Verification items for the finished model (mm, model axes). Face numbers are marked on the shaded views. A direction names the side the tool comes from. Round coordinates to 2 decimals unless told otherwise and drop trailing zeros. Order: outer loops, then holes, each group sorted by start corner. A loop starts at its lowest first (then second) coordinate and runs counter-clockwise, first axis right, second up. Notation, with made-up numbers: (51, 24.25) -> (85, 24.25) arc R38 cw to (85, 62.25) -> close; hole circle Ø3 at (81.5, 86.25). An arc over 180 degrees is marked (long way). Put each result on its own line as item: value.
```python
from build123d import *

# Parameters (mm, degrees)
SKETCH2_W          = 3.119119432
SKETCH2_H          = 0.920816202
CUT_EXTRUDE1_DEPTH = 7.874


with BuildPart() as part:
    # Sketch1 → Revolve1 (revolve)
    with BuildSketch(Plane.XY, mode=Mode.PRIVATE) as revolve1_sk:
        Polygon((0, 0), (12.7, 0), (12.7, 3.175), (1.905, 3.175), (0, 5.08), align=None)
    revolve(revolve1_sk.sketch.rotate(Axis((0, 0, 0), (1, 0, 0)), 90), axis=Axis((0, 0, 0), (1, 0, 0)))

    # Sketch2 → Cut-Extrude1 (cut, symmetric)
    with BuildSketch(Plane(origin=(0, 0, 0), x_dir=(1, 0, 0), z_dir=(0, 1, 0))):
        Rectangle(SKETCH2_W, SKETCH2_H)
    extrude(amount=CUT_EXTRUDE1_DEPTH, both=True, mode=Mode.SUBTRACT)


solid = part.part
```
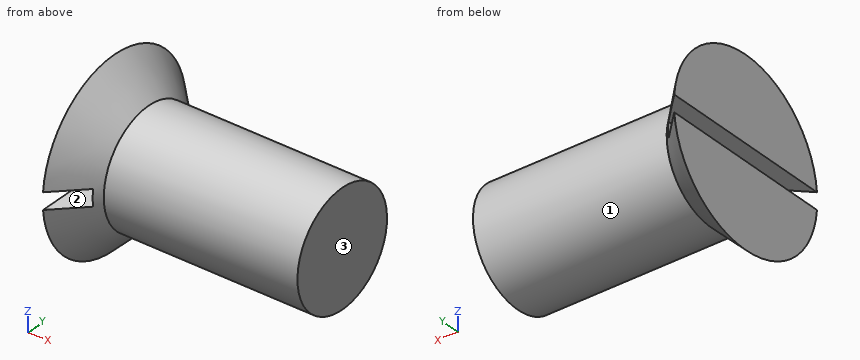
Item 1: Sectioned sample at C-C, the plane x = 1.75. Record the boundary of the cut face in (y, z), then the cut area to 3 significant figures.
Geometry check:
outline: circle Ø6.66 at (0, 0)
area: 34.8 mm2
Item 2: Tool access check on the marked faces 1, 2 and 3. Record the directions out of +Z, -Z, +X, -X, +Y, -Y that give a thin tool (end or side, any length) a straight path to the whole face; none if there is none.
Geometry check:
face 1: +X
face 2: -X, +Y, -Y
face 3: +Z, -Z, +X, +Y, -Y
Item 3: Sectioned sample at B-B, the plane z = 0. Record the boundary of the cut face in (x, y) (3 decimals), then the cut area to 3 significant figures.
Geometry check:
outline: (1.56, -3.52) -> (1.905, -3.175) -> (12.7, -3.175) -> (12.7, 3.175) -> (1.905, 3.175) -> (1.56, 3.52) -> close
area: 70.9 mm2
Item 4: Sectioned sample at A-A, the plane y = 0. Record the boundary of the cut face in (x, z) (3 decimals), then the cut area to 3 significant figures.
Geometry check:
outline: (0, -5.08) -> (1.905, -3.175) -> (12.7, -3.175) -> (12.7, 3.175) -> (1.905, 3.175) -> (0, 5.08) -> (0, 0.46) -> (1.56, 0.46) -> (1.56, -0.46) -> (0, -0.46) -> close
area: 82.8 mm2
Item 5: Depth check by flat-ended pin: pin 1 Ø0.7 at (y, z) = (-1, 0) entering from -X; pin 2 Ø1 at (x, y) = (4.5, 2.5) entering from +Z; pin 3 Ø4 at (y, z) = (1.5, -3.5) entering from -X; pin 4 Ø4 at (x, y) = (2, 1.5) entering from +Z. Enter the tip coordinate at first touch or a pass-through.
Geometry check:
pin 1: x = 1.56
pin 2: z = 2.47
pin 3: x = 0
pin 4: z = 4.92
Item 6: Sectioned sample at D-D, the plane x = 5.5. Record the boundary of the cut face in (y, z) (3 decimals), then the cut area to 3 significant figures.
Geometry check:
outline: circle Ø6.35 at (0, 0)
area: 31.7 mm2
Item 7: Material ranges on line 1 along Z through (x, y) = (0.5, 0.5); line 2 along Z through (x, y) = (0.5, -2.5); line 3 along X through (y, z) = (-2.75, -2.25), recorded low to high.
Geometry check:
line 1: -4.55 to -0.46, 0.46 to 4.55
line 2: -3.84 to -0.46, 0.46 to 3.84
line 3: 0 to 1.53
